```python
from build123d import *

# Parameters (mm, degrees)
BOSS_EXTRUDE1_DEPTH = 10
SKETCH2_R           = 1.25
CUT_EXTRUDE1_DEPTH  = 4
BOSS_EXTRUDE4_DEPTH = 10


with BuildPart() as part:
    # Sketch1 → Boss-Extrude1 (new body)
    with BuildSketch(Plane(origin=(0, 0, 0), x_dir=(0, 0, -1), z_dir=(1, 0, 0))):
        Polygon((0.362907695, 7.258153898), (-0.206723569, 7.258153898), (-6.206723569, 7.258153898), (-6.206723569, 3.258153898), (-0.637092305, 3.258153898), (-0.637092305, -12.741846102), (0.362907695, -12.741846102), align=None)
    extrude(amount=BOSS_EXTRUDE1_DEPTH)

    # Sketch2 → Cut-Extrude1 (cut)
    with BuildSketch(Plane(origin=(0, 3.258153898, 0), x_dir=(1, 0, 0), z_dir=(0, 1, 0))):
        with Locations((4.995009197, -3.206723569)):
            Circle(SKETCH2_R)
    extrude(amount=CUT_EXTRUDE1_DEPTH, mode=Mode.SUBTRACT)

    # Sketch5 → Boss-Extrude4 (add)
    with BuildSketch(Plane.ZY):
        with BuildLine():
            Line((-0.362907695, -12.741846102), (-0.362907695, 7.258153898))
            ThreePointArc((-0.362907695, 7.258153898), (-0.805423884, -2.741846102), (-0.362907695, -12.741846102))
        make_face()
    extrude(amount=-BOSS_EXTRUDE4_DEPTH)


solid = part.part
```
Can you work these out from the model? Positions are in its coordinate system, mm. A direction names the side the tool comes from. Round coordinates to 2 decimals unless told otherwise and drop trailing zeros. Loops run counter-clockwise (first coordinate to the right, second up) from the corner with the lowest first, then second, coordinate; pieces in that order, holes last. Notation, with made-up numbers: (74.25, 46) -> (89.25, 46) arc R3 cw to (89.25, 50) -> close; hole circle Ø3 at (63.5, 9). An arc over 180 degrees is marked (long way). One line per item, written item: value. Start each with the question number.
1. If we section it at A-A, the plane x = 4: Write out the boundary of the cut face in (y, z).
2. If we mould it in two halves opening along X, with no side actions, what happens to faces 1 (the flat face through (0, 0, 0)), 2 (the flat face through (5, -12.742, 0)), 3 (the cylindrical face through (6.187, 5.23, 2.831))? For each: pulls with the +X half, pulls with the -X half, needs draft (parallel to the pull), parting line crosses it, or undercut.
3. For faces 4 (the flat face through (5, -5, 0.637)), 5 (the flat face through (4, 7.258, 2)), which set-ups out of +Z, -Z, +X, -X, +Y, -Y let a thin tool reach every point of the face, with its end or its side?
4. If I drill on probe 1 along Y at (x, z) = (1.5, 1.75); probe 2 along Z at (x, y) = (9, -3.5); probe 3 along Z at (x, y) = (4.25, 5.5), over which ranges is the centre line in solid material (lowest first)?
5. For pin 1 (3 mm diameter, centred on x = 2, z = 4, fed in from -Y), with a flat end and sliding along its axis, tell me the tip position at first contact or that it passes through.
6. If we section it at D-D, the plane x = 9.25: Write out the boundary of the cut face in (y, z), then the cut area to 3 significant figures.
7. If we section it at B-B, the plane z = 4.25: Write out the boundary of the cut face in (x, y).
8. If we section it at C-C, the plane y = 5: Write out the boundary of the cut face in (x, z) (3 decimals), then the cut area to 3 significant figures.
Calculated:
1. outline: (-12.74, -0.36) arc R113.21 ccw to (7.26, -0.36) -> (7.26, 2.45) -> (3.26, 2.45) -> (3.26, 0.64) -> (-12.74, 0.64) -> close; (3.26, 3.96) -> (7.26, 3.96) -> (7.26, 6.21) -> (3.26, 6.21) -> close
2. face 1: pulls with the -X half
2. face 2: needs draft
2. face 3: undercut
3. face 4: +Z, +X, -X, -Y
3. face 5: +Z, -Z, +X, -X, +Y
4. probe 1: y = 3.26 to 7.26
4. probe 2: z = -0.8 to 0.64
4. probe 3: z = -0.51 to 2.2, 4.21 to 6.21
5. pin 1: stops at y = 3.26
6. outline: (-12.74, -0.36) arc R113.21 ccw to (7.26, -0.36) -> (7.26, 6.21) -> (3.26, 6.21) -> (3.26, 0.64) -> (-12.74, 0.64) -> close
6. area: 48.2 mm²
7. outline: (0, 3.26) -> (4.31, 3.26) -> (4.31, 7.26) -> (0, 7.26) -> close; (5.68, 3.26) -> (10, 3.26) -> (10, 7.26) -> (5.68, 7.26) -> close
8. outline: (0, -0.54) -> (10, -0.54) -> (10, 6.207) -> (0, 6.207) -> close; hole circle Ø2.5 at (4.995, 3.207)
8. area: 62.6 mm²
